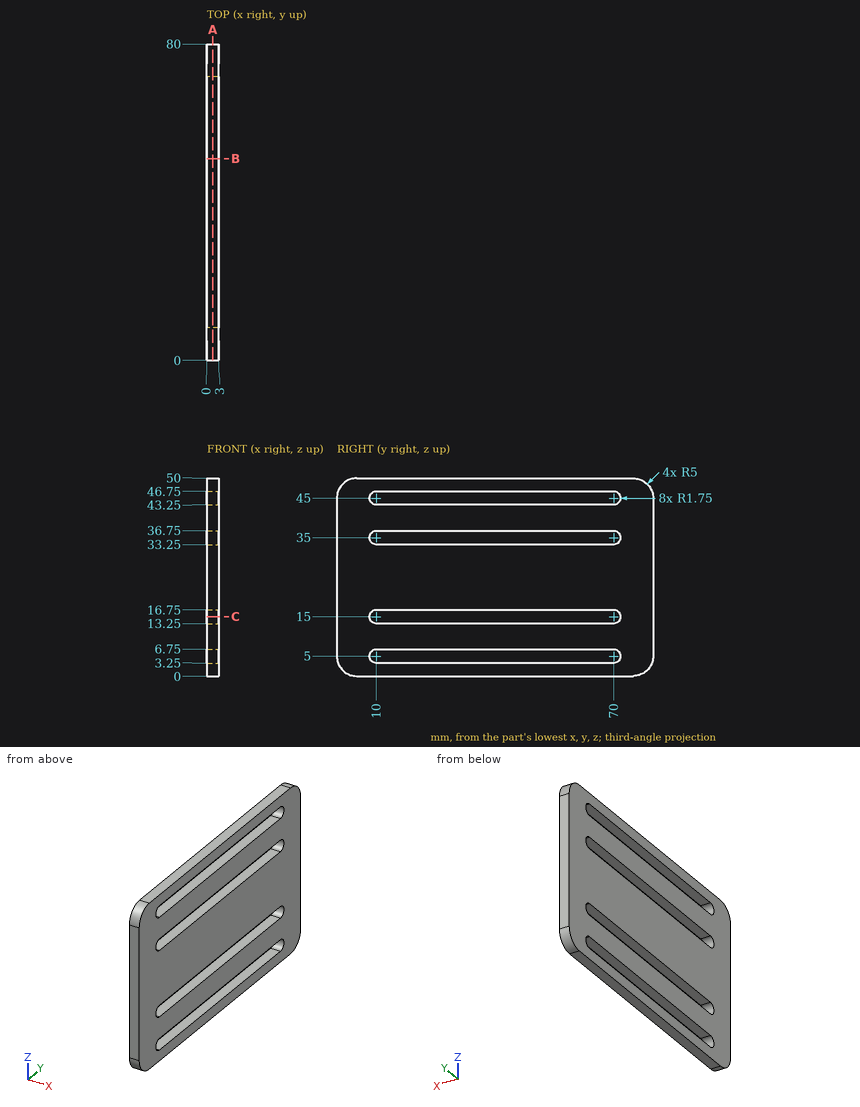
Check sheet for the drawn part. Datum: minimum x, y, z corner. Units: mm. Give positions to 0.01 mm unless a question says otherwise; leave off trailing zeros. Write each loop counter-clockwise with the first axis right and the second up, starting at its lowest first coordinate (ties: lowest second). Pieces come first, ordered by that corner, then holes.
(1) Cross-section at B-B (y = 51). Enter the section's corners in (x, z), plus the area to 3 significant figures.
(2) Cross-section at A-A (x = 1.5). Enter the section's corners in (y, z).
(3) Material ranges on line 1 (Z direction, x = 1.8, y = 24.5); line 2 (Z direction, x = 2.5, y = 8.5); line 3 (Y direction, x = 0.3, z = 36), recorded low to high.
(4) Cross-section at C-C (z = 15). Enter the section's corners in (x, y).
Worked out:
1. outline: (0, 0) - (3, 0) - (3, 3.25) - (0, 3.25) - close; (0, 6.75) - (3, 6.75) - (3, 13.25) - (0, 13.25) - close; (0, 16.75) - (3, 16.75) - (3, 33.25) - (0, 33.25) - close; (0, 36.75) - (3, 36.75) - (3, 43.25) - (0, 43.25) - close; (0, 46.75) - (3, 46.75) - (3, 50) - (0, 50) - close
1. area: 108 mm2
2. outline: (0, 5) arc R5 ccw to (5, 0) - (75, 0) arc R5 ccw to (80, 5) - (80, 45) arc R5 ccw to (75, 50) - (5, 50) arc R5 ccw to (0, 45) - close; hole (10, 3.25) - (70, 3.25) arc R1.75 ccw to (70, 6.75) - (10, 6.75) arc R1.75 ccw to start; hole (10, 13.25) - (70, 13.25) arc R1.75 ccw to (70, 16.75) - (10, 16.75) arc R1.75 ccw to start; hole (10, 33.25) - (70, 33.25) arc R1.75 ccw to (70, 36.75) - (10, 36.75) arc R1.75 ccw to start; hole (10, 43.25) - (70, 43.25) arc R1.75 ccw to (70, 46.75) - (10, 46.75) arc R1.75 ccw to start
3. line 1: z = 0 to 3.25, 6.75 to 13.25, 16.75 to 33.25, 36.75 to 43.25, 46.75 to 50
3. line 2: z = 0 to 4.1, 5.9 to 14.1, 15.9 to 34.1, 35.9 to 44.1, 45.9 to 50
3. line 3: y = 0 to 8.56, 71.44 to 80
4. outline: (0, 0) - (3, 0) - (3, 8.25) - (0, 8.25) - close; (0, 71.75) - (3, 71.75) - (3, 80) - (0, 80) - close
